Can you work these out from the model? Positions are in its coordinate system, mm. Face numbers are marked on the shaded views. Round coordinates to 2 decimals unless told otherwise and drop trailing zeros. Write each loop counter-clockwise with the first axis right and the second up, starting at its lowest first coordinate (ties: lowest second). Pieces come first, ordered by that corner, then holes. Notation, with made-up numbers: (-9.5, 85.25) - (41.5, 85.25) arc R29 cw to (41.5, 113.25) - close; hole circle Ø11 at (10.25, 21.25). An arc over 180 degrees is marked (long way). One line per item, written item: value. Start each with the question number.
(1) If I drill on L1, parallel to Z at x = 0, y = 8.9; L2, parallel to Y at x = -5, z = -9; L3, parallel to X at y = 15.75, z = 25.5, over which ranges is the centre line in solid material (lowest first)? Write a range as from..to.
(2) I'm going to push flat-ended pins straight in: pin 1 Ø8 at (y, z) = (5, 22.5) entering from -X; pin 2 Ø2 at (x, z) = (-8, 15) entering from +Y; pin 3 Ø6 at (x, y) = (15.5, 8.5) entering from -Z; pin 4 Ø1 at (x, z) = (12, -11.5) entering from -Y. Where does each tip first touch, or does it pass through?
(3) I want a section at A-A on y = 8.5. List the corners of the cut face in (x, z) for me, plus the area to 3 significant figures.
(4) Thinking about a two-plate mould opening in Z: for the marked faces 1, 2 and 3, which applies, +Z half, -Z half, draft (parallel to the pull), parting line (faces both ways), or undercut?
Autodesk Inventor part; units mm, degrees
ref_plane "YZ Plane" through (0, 0, 0) normal (1, 0, 0) x (0, 1, 0)
ref_plane "XZ Plane" through (0, 0, 0) normal (0, 1, 0) x (-1, 0, 0)
ref_plane "XY Plane" through (0, 0, 0) normal (0, 0, 1) x (1, 0, 0)
sketch "Skizze1" plane through (0, 0, 0) normal (0, 1, 0) x (-1, 0, 0)
  circle A0 centre (0, 0) radius 37
  dimension "d0" = 74
extrude "Extrusion1" add sketch "Skizze1" along normal blind 20.5
sketch "Skizze2" plane through (0, 20.5, 0) normal (0, 1, 0) x (1, 0, 0)
  circle A0 centre (0, 0) radius 30.5
  dimension "d3" = 61
extrude "Extrusion2" cut sketch "Skizze2" against normal blind 13
chamfer "Fase1" distance 5 angle 45 1 edges at (-30.5, 20.5, 0)
chamfer "Fase2" distance 5 angle 45 1 edges at (-30.5, 15.5, 0)
fillet "Rundung2" radius 1 2 edges at (37, 20.5, 0) (-35.5, 20.5, 0)
fillet "Rundung3" radius 1 2 edges at (-34.0355, 19.0355, 0) (-30.5, 10.5, 0)
properties part number "bat" material "ABS-Kunststoff"
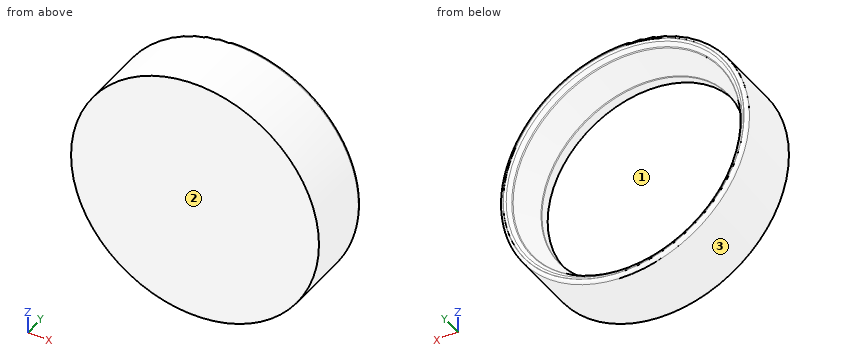
Established:
1. L1: -37..-30.5, 30.5..37
1. L2: 0..7.5
1. L3: -26.81..-20.43, 20.43..26.81
2. pin 1: x = -32.04
2. pin 2: y = 7.5
2. pin 3: z = -34.82
2. pin 4: y = 0
3. outline: circle Ø74 at (0, 0); hole circle Ø61 at (0, 0)
3. area: 1,380 mm2
4. face 1: undercut
4. face 2: draft
4. face 3: parting line
